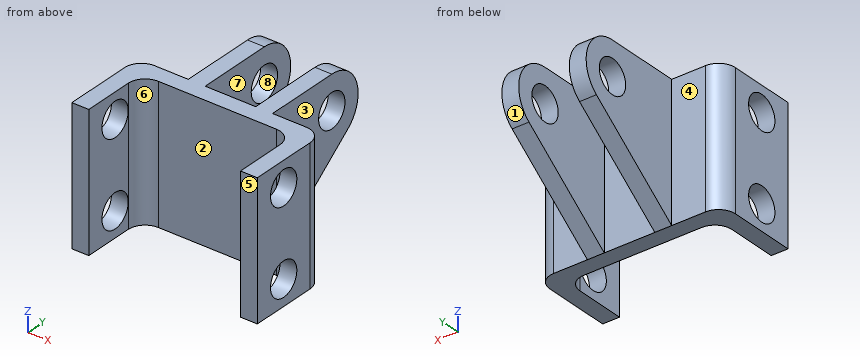
```python
from build123d import *

# Parameters (mm, degrees)
SKETCH1_R                = 10
BOSS_EXTRUDE1_DEPTH      = 10
BOSS_EXTRUDE2_DEPTH      = 25
BOSS_EXTRUDE2_DEPTH_BACK = 30
SKETCH1_4_W              = 80.000017133
SKETCH1_4_H              = 10.000013225
BOSS_EXTRUDE3_START      = -30
SKETCH1_5_W              = 80.000017133
SKETCH1_5_H              = 40
SKETCH1_5_R              = 10
BOSS_EXTRUDE3_DEPTH      = 10
FILLET1_R                = 10


with BuildPart() as part:
    # Sketch1 → Boss-Extrude1 (new body)
    with BuildSketch(Plane(origin=(0, 0, 0), x_dir=(0, 0, -1), z_dir=(1, 0, 0))):
        with BuildLine():
            Line((0, 10.000013225), (0, 55))
            ThreePointArc((0, 55), (13.54409483, 73.929376335), (35.832128843, 67.220625855))
            Line((35.832128843, 67.220625855), (80.000017133, 10.000013225))
            Line((80.000017133, 10.000013225), (0, 10.000013225))
        make_face()
        with Locations((20, 55)):
            Circle(SKETCH1_R, mode=Mode.SUBTRACT)
    extrude(amount=BOSS_EXTRUDE1_DEPTH)

    # Sketch1_4 → Boss-Extrude2 (add, two sides: drawn at the far end of the back side and taken through both)
    with BuildSketch(Plane(origin=(0, 0, 0), x_dir=(0, 0, -1), z_dir=(1, 0, 0)).offset(-BOSS_EXTRUDE2_DEPTH_BACK)):
        with Locations((40.000008567, 5.000006613)):
            Rectangle(SKETCH1_4_W, SKETCH1_4_H)
    extrude(amount=BOSS_EXTRUDE2_DEPTH + BOSS_EXTRUDE2_DEPTH_BACK)

    # Sketch1_5 → Boss-Extrude3 (add)
    with BuildSketch(Plane(origin=(0, 0, 0), x_dir=(0, 0, -1), z_dir=(1, 0, 0)).offset(BOSS_EXTRUDE3_START)):
        with Locations((40.000008567, -20)):
            Rectangle(SKETCH1_5_W, SKETCH1_5_H)
        with Locations((15, -20)):
            Circle(SKETCH1_5_R, mode=Mode.SUBTRACT)
        with Locations((65, -20)):
            Circle(SKETCH1_5_R, mode=Mode.SUBTRACT)
    extrude(amount=BOSS_EXTRUDE3_DEPTH)

    # Mirror3: part across plane


with BuildPart() as part_1:
    add(part.part)
    add(part.part.mirror(Plane(origin=(25, 0, 0), x_dir=(0, 0, 1), z_dir=(1, 0, 0))))

    # Fillet1
    fillet1_edges = [part_1.edges().sort_by_distance(p)[0] for p in [
        (70, 0, -40.000008566),
        (-20, 0, -40.000008566),
        (80, 10.000013225, -40.000008566),
        (-30, 10.000013225, -40.000008566),
    ]]
    fillet(fillet1_edges, radius=FILLET1_R)


solid = part_1.part
```
Source: CAD feature listing. Evaluate the final solid. Frame: model axes, mm. Face numbers are marked on the shaded views. A direction names the side the tool comes from. Round coordinates to 2 decimals unless told otherwise and drop trailing zeros. Write each loop counter-clockwise with the first axis right and the second up, starting at its lowest first coordinate (ties: lowest second). Pieces come first, ordered by that corner, then holes. Notation, with made-up numbers: M -18,-32.75 L 20,-32.75 A28 ccw 20,0.25 Z; hole C 61,59.5 d8. An arc over 180 degrees is marked long. Answer as a JSON object with one key per item and string values. Group by question number.
(1) Mould query, pull axis X, two halves, no side actions, for the marked faces 1, 2 and 3. Classes: +X half, -X half, draft (parallel to the pull), parting line (faces both ways), or undercut.
(2) Section query A-A on y = -20. Output: boundary loops of the cut face in (x, z), then the cut area to 3 significant figures.
(3) Reachability of the marked faces 4, 5, 6, 7 and 8 from +Z, -Z, +X, -X, +Y, -Y: full face, straight path, thin tool, end or side. Return the list, or none.
(4) Section query D-D on y = 6. Output: boundary loops of the cut face in (x, z), then the cut area to 3 significant figures.
(5) Section query C-C on x = 73. Output: boundary loops of the cut face in (y, z).
(6) First-contact query: pin 1 (5 mm diameter, centred on x = 16.5, z = -64.5, fed in from +Y); pin 2 (23 mm diameter, centred on y = -20, z = -65, fed in from -X); pin 3 (1.5 mm diameter, centred on x = 48.5, z = -34, fed in from -Y); pin 4 (4 mm diameter, centred on y = 3, z = -64.5, fed in from -X). Flat tips, straight axial feed; report the tip coordinate or a pass-through.
(7) Ray query, line 1 (Y direction, x = 29, z = -64.5); line 2 (Y direction, x = 44, z = -20); line 3 (Y direction, x = -24, z = -15). Return the intervals inside material, ascending. Write a range as [from, to].
(8) Section query B-B on z = -34. Output: boundary loops of the cut face in (x, y).
Computed values:
{
 "1": {"face 1": "draft", "face 2": "undercut", "face 3": "+X half"},
 "2": {"outline": "M -30,-80 L -20,-80 L -20,-75 L -30,-75 Z; M -30,-55 L -20,-55 L -20,-25 L -30,-25 Z; M -30,-5 L -20,-5 L -20,0 L -30,0 Z; M 70,-80 L 80,-80 L 80,-75 L 70,-75 Z; M 70,-55 L 80,-55 L 80,-25 L 70,-25 Z; M 70,-5 L 80,-5 L 80,0 L 70,0 Z", "area": "800 mm^2"},
 "3": {"face 4": "+Z, -Z, -X, +Y", "face 5": "+Z, -Z, +X, -X, -Y", "face 6": "+Z, -Z, -Y", "face 7": "+Z, -Z, +Y", "face 8": "+X, -X"},
 "4": {"outline": "M -28,-80 L 78,-80 L 78,0 L -28,0 Z", "area": "8,480 mm^2"},
 "5": {"outline": "M -40,-80 L 9.54,-80 L 9.54,0 L -40,0 Z; hole C -20,-65 d20; hole C -20,-15 d20"},
 "6": {"pin 1": "y = 10", "pin 2": "x = -30", "pin 3": "y = 0", "pin 4": "x = -29.95"},
 "7": {"line 1": "[0, 10]", "line 2": "[0, 45], [65, 75]", "line 3": "[-40, -30], [-10, 9.17]"},
 "8": {"outline": "M -30,-40 L -20,-40 L -20,-10 A10 cw -10,0 L 60,0 A10 cw 70,-10 L 70,-40 L 80,-40 L 80,0 A10 ccw 70,10 L 50,10 L 50,69.28 L 40,69.28 L 40,10 L 10,10 L 10,69.28 L 0,69.28 L 0,10 L -20,10 A10 ccw -30,0 Z"}
}
